Autodesk Inventor part; units mm, degrees
ref_plane "YZ Plane" through (0, 0, 0) normal (1, 0, 0) x (0, 1, 0)
ref_plane "XZ Plane" through (0, 0, 0) normal (0, 1, 0) x (-1, 0, 0)
ref_plane "XY Plane" through (0, 0, 0) normal (0, 0, 1) x (1, 0, 0)
sketch "スケッチ1" plane through (0, 0, 0) normal (1, 0, 0) x (0, 1, 0)
  circle A0 centre (0, 0) radius 5 construction
  circle A1 centre (0, 0) radius 3.6
  arc A2 (1.4444, 4.7868) -> (-1.8694, -4.6374) centre (0, 0) ccw
  line L0 (-1.8694, -4.6374) -> (0, -5.391)
  line L1 (0, -5.391) -> (0, -32.1321)
  line L2 (0, -32.1321) -> (24.603, -32.1321)
  line L3 (24.603, -32.1321) -> (24.603, -2.2012)
  line L4 (24.603, -2.2012) -> (1.4444, 4.7868)
  circle A3 centre (0, 0) radius 3
  circle A4 centre (12.3015, -20.4215) radius 1.6
  circle A5 centre (12.3015, -20.4215) radius 8 construction
  circle A6 centre (20.3015, -20.4215) radius 1.55
  line L5 (20.3015, -20.4215) -> (4.3015, -20.4215) construction
  circle A7 centre (4.3015, -20.4215) radius 1.55
  circle A8 centre (12.3015, -20.4215) radius 14 construction
  dimension "d1" = 10
  dimension "d0" = 7.2
  dimension "d4" = 6
  dimension "d7" = 3.2
  dimension "d8" = 16
  dimension "d9" = 3.1
  dimension "d10" = 28
extrude "押し出し1" add sketch "スケッチ1" along normal blind 2.5 contours A1 | L4 L3 L2 L1 L0 A2
extrude "押し出し2" cut sketch "スケッチ1" along normal blind 0.6 contours A1 | A3
properties part number "Gear_Frame"
Source: CAD feature listing. Evaluate the final solid. Frame: model axes, mm. A direction names the side the tool comes from. Coordinates: 2 decimals unless noted, no trailing zeros. Write each loop counter-clockwise with the first axis right and the second up, starting at its lowest first coordinate (ties: lowest second). Pieces come first, ordered by that corner, then holes. Notation, with made-up numbers: (58.5, 19) -> (85.5, 19) arc R36 ccw to (85.5, 53) -> close; hole circle Ø3 at (28.5, 48). An arc over 180 degrees is marked (long way). Return JSON: item names as keys, results as strings. Group by question number.
1) Ray query, line 1 along Z through (x, y) = (0.25, 3); line 2 along Y through (x, z) = (0.3, -21); line 3 along Z through (x, y) = (1.2, 9). Return the intervals inside material, ascending.
2) Section query C-C, the plane x = 1.15. Return loops of the section in (y, z), plus the area to 3 significant figures.
3) Section query B-B, the plane z = 0. Return loops of the section in (x, y), plus the area to 3 significant figures.
4) Section query D-D, the plane z = -16. Return loops of the section in (x, y).
5) Set-up query: faces 4 (the face through (1, 0, -19)), 5 (the face through (0.6, -1, 3)), 6 (the face through (1, 24.603, -17)). Return all of +Z, -Z, +X, -X, +Y, -Y with unobstructed straight access to the full face (end or side cutting, diameter ignored); none if empty.
6) Mould query, pull axis Z, two halves, no side actions, for faces 1 (the face through (2, -3, 0)), 2 (the face through (1.23, -0.95, -5.01)), 3 (the face through (1.23, -4.75, 1.56)). Classes: +Z half, -Z half, draft (parallel to the pull), parting line (faces both ways), or undercut.
7) Section query A-A, the plane y = 13. Return loops of the section in (x, z).
From the geometry:
{
 "1": {"line 1": "-32.13 to -21.26, -19.58 to -1.99, 1.99 to 4.32", "line 2": "0 to 2.86, 5.74 to 10.81, 13.79 to 18.86, 21.74 to 24.6", "line 3": "-32.13 to 2.51"},
 "2": {"outline": "(-1.87, -4.64) -> (0, -5.39) -> (0, -32.13) -> (24.6, -32.13) -> (24.6, -2.2) -> (1.44, 4.79) arc R5 ccw to start; hole circle Ø6 at (0, 0); hole circle Ø3.1 at (4.3, -20.42); hole circle Ø3.2 at (12.3, -20.42); hole circle Ø3.1 at (20.3, -20.42)", "area": "816 mm²"},
 "3": {"outline": "(0, -5) -> (2.5, -5) -> (2.5, -3) -> (0.6, -3) -> (0.6, -3.6) -> (0, -3.6) -> close; (0, 3.6) -> (0.6, 3.6) -> (0.6, 3) -> (2.5, 3) -> (2.5, 17.31) -> (0, 17.31) -> close", "area": "40.1 mm²"},
 "4": {"outline": "(0, 0) -> (2.5, 0) -> (2.5, 24.6) -> (0, 24.6) -> close"},
 "5": {"face 4": "-Z, +X, -X, -Y", "face 5": "-X", "face 6": "+Z, -Z, +X, -X, +Y"},
 "6": {"face 1": "undercut", "face 2": "-Z half", "face 3": "parting line"},
 "7": {"outline": "(0, -32.13) -> (2.5, -32.13) -> (2.5, -21.86) -> (0, -21.86) -> close; (0, -18.98) -> (2.5, -18.98) -> (2.5, 1.3) -> (0, 1.3) -> close"}
}
